The model under review builds one solid part; all positions refer to its coordinate system, in mm. Face numbers are marked on the shaded views. A direction names the side the tool comes from. Coordinates: 2 decimals unless noted, no trailing zeros. Write each loop counter-clockwise with the first axis right and the second up, starting at its lowest first coordinate (ties: lowest second). Pieces come first, ordered by that corner, then holes. Notation, with made-up numbers: (85, 17.25) - (132, 17.25) arc R10 cw to (132, 24.25) - close; hole circle Ø1 at (-25.75, 58). An arc over 180 degrees is marked (long way). Return JSON: item names as keys, results as strings. Group by question number.
(1) We need section A-A on x = 0. State the section outline as (y, z) points, then the cut area to 3 significant figures.
(2) We need section D-D on x = 10. State the section outline as (y, z) points.
(3) For pin 1 Ø1 at (y, z) = (5, -1.5) entering from -X; pin 2 Ø10 at (x, z) = (0.5, 5.5) entering from -Y; pin 3 Ø1 at (x, z) = (-3, 4.5) entering from +Y; pin 4 Ø3.5 at (x, y) = (0, 5) entering from -Z, all flat-tipped, find the tip position at first contact; note any pin that passes through.
(4) Tool access review of the marked faces 1 and 2: name each direction out of +Z, -Z, +X, -X, +Y, -Y from which nothing blocks a thin tool from reaching the whole face with its end or side.
(5) To check wall thickness, follow L1, parallel to Z at x = 3, y = 6; L2, parallel to Y at x = -7, z = -13; L3, parallel to Z at x = 6, y = 6.5. State the ranges of each line that lie inside material, in increasing order. Write a range as from..to.
(6) Draft analysis for pull direction X (two halves, no side actions). For the marked faces 3, 4, 5 and 6, state which applies: released by +X, released by -X, zero draft, split by the parting line, or undercut.
(7) We need section B-B on z = 5.5. State the section outline as (x, y) points, then the cut area to 3 significant figures.
Autodesk Inventor part; units mm, degrees
ref_plane "YZ Plane" through (0, 0, 0) normal (1, 0, 0) x (0, 1, 0)
ref_plane "XZ Plane" through (0, 0, 0) normal (0, 1, 0) x (-1, 0, 0)
ref_plane "XY Plane" through (0, 0, 0) normal (0, 0, 1) x (1, 0, 0)
sketch "Sketch1" plane through (0, 0, 0) normal (0, 1, 0) x (-1, 0, 0)
  circle A0 centre (0, 0) radius 14.2875
  line L0 (3.6662, 6.35) -> (7.3323, 0)
  line L1 (7.3323, 0) -> (3.6662, -6.35)
  line L2 (3.6662, -6.35) -> (-3.6662, -6.35)
  line L3 (-3.6662, -6.35) -> (-7.3323, 0)
  line L4 (-7.3323, 0) -> (-3.6662, 6.35)
  line L5 (-3.6662, 6.35) -> (3.6662, 6.35)
  dimension "d0" = 28.575
  dimension "d1" = 12.7
extrude "Extrusion1" add sketch "Sketch1" along normal blind 7.7724
sketch "Sketch2" plane through (0, 7.7724, 0) normal (0, 1, 0) x (1, 0, 0)
  circle A0 centre (0, 0) radius 15.5575
  line L0 (-3.6662, 6.35) -> (3.6662, 6.35)
  line L1 (-3.6662, 6.35) -> (3.6662, 6.35)
  line L2 (3.6662, 6.35) -> (7.3323, 0)
  line L3 (7.3323, 0) -> (3.6662, -6.35)
  line L4 (3.6662, -6.35) -> (-3.6662, -6.35)
  line L5 (-3.6662, -6.35) -> (-7.3323, 0)
  line L6 (-7.3323, 0) -> (-3.6662, 6.35)
  dimension "d4" = 31.115
extrude "Extrusion2" add sketch "Sketch2" along normal blind 1.524
properties part number "hex bearing" material "Steel"
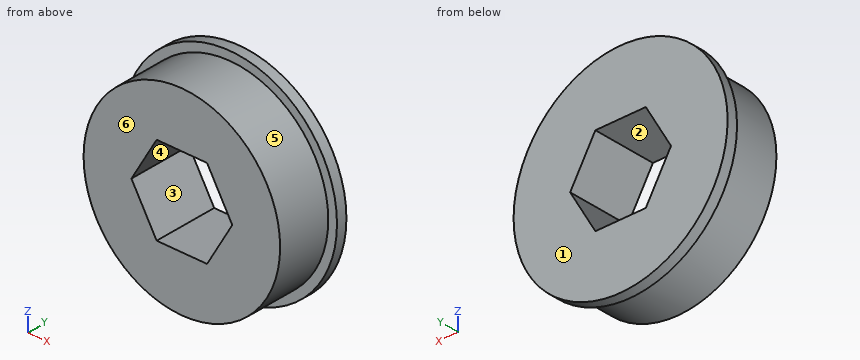
Ans:
{
 "1": {"outline": "(0, -14.29) - (7.77, -14.29) - (7.77, -15.56) - (9.3, -15.56) - (9.3, -6.35) - (0, -6.35) - close; (0, 6.35) - (9.3, 6.35) - (9.3, 15.56) - (7.77, 15.56) - (7.77, 14.29) - (0, 14.29) - close", "area": "151 mm²"},
 "2": {"outline": "(0, -10.2) - (7.77, -10.2) - (7.77, -11.92) - (9.3, -11.92) - (9.3, 11.92) - (7.77, 11.92) - (7.77, 10.2) - (0, 10.2) - close"},
 "3": {"pin 1": "x = -14.25", "pin 2": "y = 0", "pin 3": "through", "pin 4": "z = -14.29"},
 "4": {"face 1": "+Z, -Z, +X, -X, +Y", "face 2": "+Y, -Y"},
 "5": {"L1": "-13.97..-6.35, 6.35..13.97", "L2": "7.77..9.3", "L3": "-12.97..-2.31, 2.31..12.97"},
 "6": {"face 3": "undercut", "face 4": "undercut", "face 5": "split by the parting line", "face 6": "zero draft"},
 "7": {"outline": "(-14.55, 7.77) - (-13.19, 7.77) - (-13.19, 0) - (-4.16, 0) - (-4.16, 9.3) - (-14.55, 9.3) - close; (4.16, 0) - (13.19, 0) - (13.19, 7.77) - (14.55, 7.77) - (14.55, 9.3) - (4.16, 9.3) - close", "area": "172 mm²"}
}
